Verification items for this drawing (mm, ordinates from the low corner). Round coordinates to 2 decimals unless told otherwise and drop trailing zeros. Write each loop counter-clockwise with the first axis right and the second up, starting at its lowest first coordinate (ties: lowest second). Pieces come first, ordered by that corner, then holes.
Item 1: Scan lines: probe 1 along Z at (x, y) = (31.75, 3.5) (1 decimal); probe 2 along X at (y, z) = (13.5, 39.5) (1 decimal); probe 3 along X at (y, z) = (9, 43) (1 decimal). Record each from-to range of solid material in increasing order.
Item 2: Cross-section at A-A (y = 5.25). Enter the section's corners in (x, z).
Item 3: Cross-section at B-B (z = 56). Enter the section's corners in (x, y).
Item 4: Depth check by flat-ended pin: P1, Ø4, axis at x = 31.75, z = 31.75, coming from the -Y side; P2, Ø4, axis at y = 4, z = 65.5, coming from the -X side; P3, Ø10, axis at y = 8.5, z = 74, coming from the +X side. Enter the tip coordinate at first touch or a pass-through.
Item 5: Cross-section at C-C (z = 73.5). Enter the section's corners in (x, y).
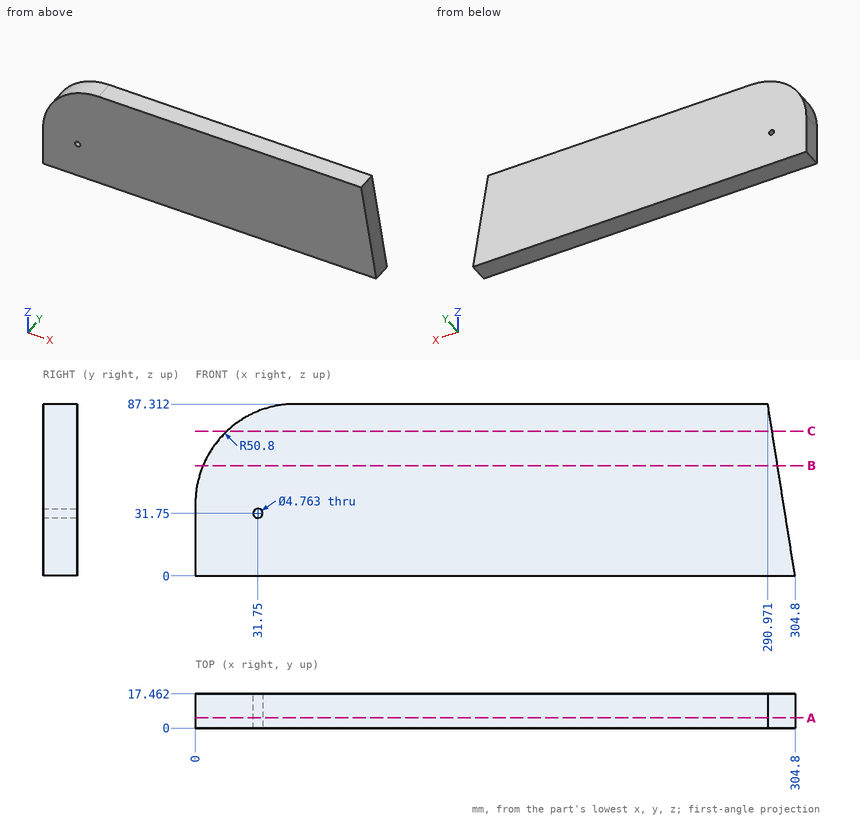
Resolved:
1. probe 1: z = 0 to 29.4, 34.1 to 83.6
1. probe 2: x = 0.1 to 298.5
1. probe 3: x = 0.4 to 298
2. outline: (0, 0) - (304.8, 0) - (290.97, 87.31) - (50.8, 87.31) arc R50.8 ccw to (0, 36.51) - close; hole circle Ø4.76 at (31.75, 31.75)
3. outline: (3.89, 0) - (295.93, 0) - (295.93, 17.46) - (3.89, 17.46) - close
4. P1: passes through
4. P2: stops at x = 7.76
4. P3: stops at x = 293.87
5. outline: (15.98, 0) - (293.16, 0) - (293.16, 17.46) - (15.98, 17.46) - close
